from build123d import *

# Parameters (mm, degrees)
EXTRUDE_1_DEPTH          = 2.5
FILLET_1_R               = 10
FILLET_2_R               = 10
FILLET_3_R               = 10
FILLET_4_R               = 10
SKETCH_2_R               = 5
SKETCH_2_R_2             = 1.52
SKETCH_2_W               = 15
SKETCH_2_H               = 2.887641603
CUT_EXTRUDE_1_DEPTH      = 49
FILLET_5_R               = 20
FILLET_6_R               = 20
PATTERN_CIRCULAR_2_COUNT = 4
SKETCH_3_R               = 6
CUT_EXTRUDE_2_DEPTH      = 49
FILLET_7_R               = 20
FILLET_8_R               = 20
FILLET_9_R               = 20
FILLET_10_R              = 20
FILLET_11_R              = 20
FILLET_12_R              = 20
SKETCH_6_W               = 24
SKETCH_6_H               = 5
SKETCH_6_W_2             = 5
SKETCH_6_H_2             = 24
EXTRUDE_2_DEPTH          = 7.5
SKETCH_7_R               = 1.52
CUT_EXTRUDE_4_DEPTH      = 16
SKETCH_8_R               = 4
CUT_EXTRUDE_5_DEPTH      = 57
FILLET_13_R              = 5
FILLET_14_R              = 5
FILLET_15_R              = 5
FILLET_16_R              = 5
FILLET_17_R              = 5
FILLET_18_R              = 5
FILLET_19_R              = 5
FILLET_20_R              = 5
SKETCH_9_R               = 4.001458819
CUT_EXTRUDE_6_DEPTH      = 57
SKETCH_10_R              = 1.52
CUT_EXTRUDE_7_DEPTH      = 57


with BuildPart() as part:
    # 草图1 → 凸台-拉伸1 (new body)
    with BuildSketch(Plane(origin=(0, 0, 0), x_dir=(1, 0, 0), z_dir=(0, 1, 0))):
        with BuildLine():
            Line((31.819805153, -31.819805153), (15.840551385, -31.819805153))
            ThreePointArc((15.840551385, -31.819805153), (0, -28.683478044), (-15.840551385, -31.819805153))
            Line((-15.840551385, -31.819805153), (-31.819805153, -31.819805153))
            Line((-31.819805153, -31.819805153), (-31.819805153, -15.840551385))
            ThreePointArc((-31.819805153, -15.840551385), (-28.683478044, 0), (-31.819805153, 15.840551385))
            Line((-31.819805153, 15.840551385), (-31.819805153, 31.819805153))
            Line((-31.819805153, 31.819805153), (-15.840551385, 31.819805153))
            ThreePointArc((-15.840551385, 31.819805153), (0, 28.683478044), (15.840551385, 31.819805153))
            Line((15.840551385, 31.819805153), (31.819805153, 31.819805153))
            Line((31.819805153, 31.819805153), (31.819805153, 15.840551385))
            ThreePointArc((31.819805153, 15.840551385), (28.683478044, 0), (31.819805153, -15.840551385))
            Line((31.819805153, -15.840551385), (31.819805153, -31.819805153))
        make_face()
    extrude(amount=EXTRUDE_1_DEPTH)

    # 圆角1
    fillet_1_edges = [part.edges().sort_by_distance(p)[0] for p in [
        (31.819805153, 1.25, 31.819805153),
    ]]
    fillet(fillet_1_edges, radius=FILLET_1_R)

    # 圆角2
    fillet_2_edges = [part.edges().sort_by_distance(p)[0] for p in [
        (31.819805153, 1.25, -31.819805153),
    ]]
    fillet(fillet_2_edges, radius=FILLET_2_R)

    # 圆角3
    fillet_3_edges = [part.edges().sort_by_distance(p)[0] for p in [
        (-31.819805153, 1.25, -31.819805153),
    ]]
    fillet(fillet_3_edges, radius=FILLET_3_R)

    # 圆角4
    fillet_4_edges = [part.edges().sort_by_distance(p)[0] for p in [
        (-31.819805153, 1.25, 31.819805153),
    ]]
    fillet(fillet_4_edges, radius=FILLET_4_R)

    # 草图2 → 切除-拉伸1 (cut)
    with BuildSketch(Plane(origin=(0, 2.5, 0), x_dir=(1, 0, 0), z_dir=(0, 1, 0))):
        with Locations(Location((-20.387793681, 20.387793681, 0), (0, 0, 270))):
            Circle(SKETCH_2_R)
        with Locations((-46.88466688, 53.955734692)):
            Circle(SKETCH_2_R_2)
        with Locations((-53.955734692, 46.88466688)):
            Circle(SKETCH_2_R_2)
        with Locations((0, 13.350698667)):
            Rectangle(SKETCH_2_W, SKETCH_2_H)
    cut_extrude_1 = extrude(amount=-CUT_EXTRUDE_1_DEPTH, mode=Mode.SUBTRACT)

    # 圆角5
    fillet_5_edges = [part.edges().sort_by_distance(p)[0] for p in [
        (-15.840551385, 1.25, -31.819805153),
    ]]
    fillet(fillet_5_edges, radius=FILLET_5_R)

    # 圆角6
    fillet_6_edges = [part.edges().sort_by_distance(p)[0] for p in [
        (-31.819805153, 1.25, -15.840551385),
    ]]
    fillet(fillet_6_edges, radius=FILLET_6_R)

    # 阵列(圆周)2: 切除-拉伸1 ×4 about axis
    pattern_circular_2_axis = Axis((0, 0, 0), (0, 1, 0))
    for i in range(1, PATTERN_CIRCULAR_2_COUNT):
        add(cut_extrude_1.rotate(pattern_circular_2_axis, i * 360 / PATTERN_CIRCULAR_2_COUNT), mode=Mode.SUBTRACT)

    # 草图3 → 切除-拉伸2 (cut)
    with BuildSketch(Plane(origin=(0, 2.5, 0), x_dir=(1, 0, 0), z_dir=(0, 1, 0))):
        with Locations(Location((0, 0, 0), (0, 0, 270))):
            Circle(SKETCH_3_R)
    extrude(amount=-CUT_EXTRUDE_2_DEPTH, mode=Mode.SUBTRACT)

    # 圆角7
    fillet_7_edges = [part.edges().sort_by_distance(p)[0] for p in [
        (31.819805153, 1.25, 15.840551385),
    ]]
    fillet(fillet_7_edges, radius=FILLET_7_R)

    # 圆角8
    fillet_8_edges = [part.edges().sort_by_distance(p)[0] for p in [
        (15.840551385, 1.25, 31.819805153),
    ]]
    fillet(fillet_8_edges, radius=FILLET_8_R)

    # 圆角9
    fillet_9_edges = [part.edges().sort_by_distance(p)[0] for p in [
        (-31.819805153, 1.25, 15.840551385),
    ]]
    fillet(fillet_9_edges, radius=FILLET_9_R)

    # 圆角10
    fillet_10_edges = [part.edges().sort_by_distance(p)[0] for p in [
        (-15.840551385, 1.25, 31.819805153),
    ]]
    fillet(fillet_10_edges, radius=FILLET_10_R)

    # 圆角11
    fillet_11_edges = [part.edges().sort_by_distance(p)[0] for p in [
        (15.840551385, 1.25, -31.819805153),
    ]]
    fillet(fillet_11_edges, radius=FILLET_11_R)

    # 圆角12
    fillet_12_edges = [part.edges().sort_by_distance(p)[0] for p in [
        (31.819805153, 1.25, -15.840551385),
    ]]
    fillet(fillet_12_edges, radius=FILLET_12_R)

    # 草图6 → 凸台-拉伸2 (add)
    with BuildSketch(Plane(origin=(0, 2.5, 0), x_dir=(1, 0, 0), z_dir=(0, 1, 0))):
        with Locations((0, 22)):
            Rectangle(SKETCH_6_W, SKETCH_6_H)
        with Locations((22, 0)):
            Rectangle(SKETCH_6_W_2, SKETCH_6_H_2)
        with Locations((0, -22)):
            Rectangle(SKETCH_6_W, SKETCH_6_H)
        with Locations((-22, 0)):
            Rectangle(SKETCH_6_W_2, SKETCH_6_H_2)
    extrude(amount=EXTRUDE_2_DEPTH)

    # 草图7 → 切除-拉伸4 (cut)
    with BuildSketch(Plane.XZ):
        with Locations(Location((-22, 0, 0), (0, 0, 270))):
            Circle(SKETCH_7_R)
        with Locations(Location((22, 0, 0), (0, 0, 270))):
            Circle(SKETCH_7_R)
        with Locations(Location((-8, 22, 0), (0, 0, 270))):
            Circle(SKETCH_7_R)
        with Locations(Location((8, 22, 0), (0, 0, 90))):
            Circle(SKETCH_7_R)
        with Locations(Location((-8, -22, 0), (0, 0, 270))):
            Circle(SKETCH_7_R)
        with Locations(Location((8, -22, 0), (0, 0, 270))):
            Circle(SKETCH_7_R)
    extrude(amount=-CUT_EXTRUDE_4_DEPTH, mode=Mode.SUBTRACT)

    # 草图8 → 切除-拉伸5 (cut)
    with BuildSketch(Plane(origin=(0, 0, -24.5), x_dir=(-1, 0, 0), z_dir=(0, 0, -1))):
        with Locations((0, 10)):
            Circle(SKETCH_8_R)
    extrude(amount=-CUT_EXTRUDE_5_DEPTH, mode=Mode.SUBTRACT)

    # 圆角13
    # the kernel refuses this fillet: 5 mm, written as the material it takes off along each edge
    with BuildSketch(Plane(origin=(-4, 10, 10.791713066), x_dir=(-1, 0, 0), z_dir=(0, 0, 1))) as fillet_13_piece_1:
        with BuildLine():
            CenterArc((3.483314774, 5), FILLET_13_R, 213.748988596, 56.251011404)
            ThreePointArc((-0.674082323, 2.222222222), (-0.172228409, 1.161104925), (0, 0))
            Line((0, 0), (3.483314774, 0))
        make_face()
    extrude(amount=22.416573868, mode=Mode.SUBTRACT)

    # 圆角14
    # the kernel refuses this fillet: 5 mm, written as the material it takes off along each edge
    with BuildSketch(Plane(origin=(4, 10, 33.208286934), x_dir=(1, 0, 0), z_dir=(0, 0, -1))) as fillet_14_piece_1:
        with BuildLine():
            CenterArc((3.483314774, 5), FILLET_14_R, 213.748988596, 56.251011404)
            ThreePointArc((-0.674082323, 2.222222222), (-0.172228409, 1.161104925), (0, 0))
            Line((0, 0), (3.483314774, 0))
        make_face()
    extrude(amount=22.416573868, mode=Mode.SUBTRACT)

    # 圆角15
    # the kernel refuses this fillet: 5 mm, written as the material it takes off along each edge
    with BuildSketch(Plane(origin=(-4, 10, -33.208286934), x_dir=(-1, 0, 0), z_dir=(0, 0, 1))) as fillet_15_piece_1:
        with BuildLine():
            CenterArc((3.483314774, 5), FILLET_15_R, 213.748988596, 56.251011404)
            ThreePointArc((-0.674082323, 2.222222222), (-0.172228409, 1.161104925), (0, 0))
            Line((0, 0), (3.483314774, 0))
        make_face()
    extrude(amount=22.416573868, mode=Mode.SUBTRACT)

    # 圆角16
    # the kernel refuses this fillet: 5 mm, written as the material it takes off along each edge
    with BuildSketch(Plane(origin=(4, 10, -10.791713066), x_dir=(1, 0, 0), z_dir=(0, 0, -1))) as fillet_16_piece_1:
        with BuildLine():
            CenterArc((3.483314774, 5), FILLET_16_R, 213.748988596, 56.251011404)
            ThreePointArc((-0.674082323, 2.222222222), (-0.172228409, 1.161104925), (0, 0))
            Line((0, 0), (3.483314774, 0))
        make_face()
    extrude(amount=22.416573868, mode=Mode.SUBTRACT)

    # 圆角17
    fillet_17_edges = [part.edges().sort_by_distance(p)[0] for p in [
        (-22, 10, -12),
    ]]
    fillet(fillet_17_edges, radius=FILLET_17_R)

    # 圆角18
    fillet_18_edges = [part.edges().sort_by_distance(p)[0] for p in [
        (-22, 10, 12),
    ]]
    fillet(fillet_18_edges, radius=FILLET_18_R)

    # 圆角19
    fillet_19_edges = [part.edges().sort_by_distance(p)[0] for p in [
        (22, 10, 12),
    ]]
    fillet(fillet_19_edges, radius=FILLET_19_R)

    # 圆角20
    fillet_20_edges = [part.edges().sort_by_distance(p)[0] for p in [
        (22, 10, -12),
    ]]
    fillet(fillet_20_edges, radius=FILLET_20_R)

    # 草图9 → 切除-拉伸6 (cut)
    with BuildSketch(Plane(origin=(24.5, 0, 0), x_dir=(0, 0, -1), z_dir=(1, 0, 0))):
        with Locations((11.758178517, 6.536143614)):
            Circle(SKETCH_9_R)
        with Locations((-11.758178517, 6.536143614)):
            Circle(SKETCH_9_R)
    extrude(amount=-CUT_EXTRUDE_6_DEPTH, mode=Mode.SUBTRACT)

    # 草图10 → 切除-拉伸7 (cut)
    with BuildSketch(Plane.ZY.offset(24.5)):
        with Locations((-5, 6.25)):
            Circle(SKETCH_10_R)
        with Locations((5, 6.25)):
            Circle(SKETCH_10_R)
    extrude(amount=-CUT_EXTRUDE_7_DEPTH, mode=Mode.SUBTRACT)


solid = part.part
Here's how the part is built. I have some questions about the finished solid (model axes, mm). A direction names the side the tool comes from. Give positions to 0.01 mm unless a question says otherwise; leave off trailing zeros. Order: outer loops, then holes, each group sorted by start corner. A loop starts at its lowest first (then second) coordinate and runs counter-clockwise, first axis right, second up. Notation, with made-up numbers: (64, 16.5) -> (93, 16.5) arc R9 ccw to (93, 32.5) -> close; hole circle Ø4 at (-35.75, 88.25). An arc over 180 degrees is marked (long way). One line per item, written item: value. Start each with the question number.
1. Will these pins go through, and if not, where does the flat tip stop? pin 1 Ø2 at (y, z) = (1.5, -3) entering from +X; pin 2 Ø4 at (x, y) = (-5, 2.5) entering from -Z; pin 3 Ø1 at (y, z) = (9, 4) entering from -X.
2. We'd pull the mould along X, two halves only. Please class faces 1 (the face through (-31.57, 1.27, -16.25)), 2 (the face through (0, 1, 11.907)), 3 (the face through (22.035, 9.885, -8.064)): released by +X, released by -X, zero draft, split by the parting line, or undercut.
3. Imagine slicing it at B-B, the plane z = 0. Count the separate pieces of the cut face and the enclosed holes in it, plus the area to 3 significant figures.
4. Imagine slicing it at A-A, the plane x = 0. List the corners of the cut face in (y, z) for me.
5. Imagine slicing it at C-C, the plane x = 17. List the corners of the cut face in (y, z) for me, plus the area to 3 significant figures.
6. For faces 4 (the face through (-14.795, 1, 0)), 5 (the face through (-12, 6, -22)), 6 (the face through (-19.5, 6, 0)), which set-ups out of +Z, -Z, +X, -X, +Y, -Y let a thin tool reach every point of the face, with its end or its side?
7. I need wall thicknesses on probe 1 along X at (y, z) = (6.5, 0); probe 2 along X at (y, z) = (4.5, 22); probe 3 along Z at (x, y) = (20, 1.25). Which ranges of each line are inside material? Lowest first, please. Write a range as from..to.
8. Imagine slicing it at D-D, the plane z = -10.5. List the corners of the cut face in (x, y) for me.
Values follow:
1. pin 1: stops at x = 28.88
1. pin 2: stops at z = -29.28
1. pin 3: stops at x = -24.5
2. face 1: released by -X
2. face 2: undercut
2. face 3: zero draft
3. separate pieces: 6
3. enclosed holes: 0
3. area: 113 mm2
4. outline: (0, -28.68) -> (2.5, -28.68) -> (2.5, -24.5) -> (6, -24.5) -> (6, -19.5) -> (2.5, -19.5) -> (2.5, -14.79) -> (0, -14.79) -> close; (0, -11.91) -> (2.5, -11.91) -> (2.5, -6) -> (0, -6) -> close; (0, 6) -> (2.5, 6) -> (2.5, 11.91) -> (0, 11.91) -> close; (0, 14.79) -> (2.5, 14.79) -> (2.5, 19.5) -> (6, 19.5) -> (6, 24.5) -> (2.5, 24.5) -> (2.5, 28.68) -> (0, 28.68) -> close
5. outline: (0, -31.68) -> (2.5, -31.68) -> (2.5, -24.07) -> (0, -24.07) -> close; (0, -16.71) -> (2.5, -16.71) -> (2.5, 16.71) -> (0, 16.71) -> close; (0, 24.07) -> (2.5, 24.07) -> (2.5, 31.68) -> (0, 31.68) -> close
5. area: 122 mm2
6. face 4: +Y, -Y
6. face 5: +Z, -Z, -X, +Y
6. face 6: +Z, -Z, +Y
7. probe 1: x = -24.5..-23.52, -20.48..-19.5, 19.5..20.48, 23.52..24.5
7. probe 2: x = -12..-9.52, -6.48..6.48, 9.52..12
7. probe 3: z = -31.82..-25.37, -15.4..15.4, 25.37..31.82
8. outline: (-30.03, 0) -> (30.03, 0) -> (30.03, 2.5) -> (24.5, 2.5) -> (24.5, 2.74) -> (19.5, 2.74) -> (19.5, 2.5) -> (-19.5, 2.5) -> (-19.5, 2.74) -> (-24.5, 2.74) -> (-24.5, 2.5) -> (-30.03, 2.5) -> close
